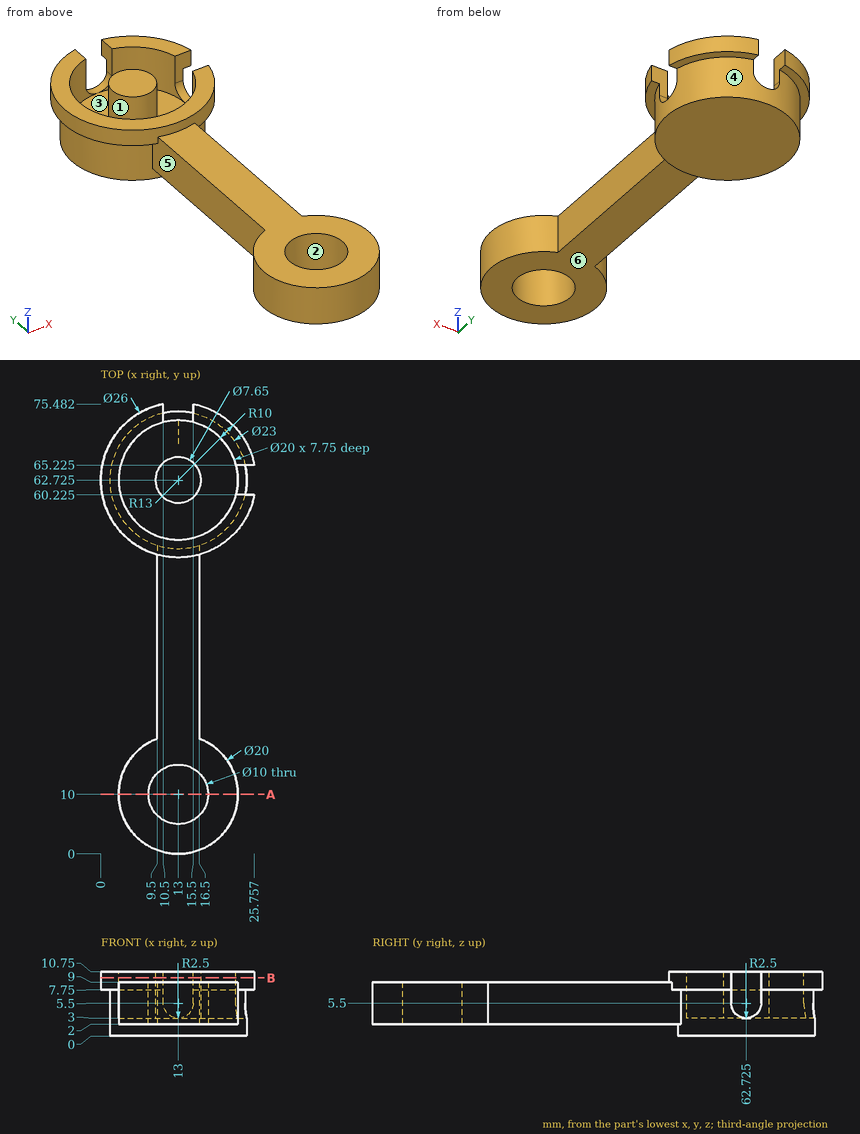
Input: dimensioned drawing with shaded views. Units: mm. Origin: part minimum x, y, z. A direction names the side the tool comes from. Give positions to 0.01 mm unless a question says otherwise; leave off trailing zeros. Write each loop counter-clockwise with the first axis right and the second up, starting at its lowest first coordinate (ties: lowest second). Pieces come first, ordered by that corner, then holes. Notation, with made-up numbers: (4, 88.25) - (52, 88.25) arc R15 ccw to (52, 109.25) - close; hole circle Ø2 at (60, 68). An arc over 180 degrees is marked (long way). One line per item, written item: value. Start each with the question number.
Q1. Material intervals for probe 1 along Y at (x, z) = (4.5, 4.75) (1 decimal); probe 2 along X at (y, z) = (28, 4); probe 3 along Y at (x, z) = (11, 4.5) (1 decimal), sorted ascending. Write a range as from..to.
Q2. First-contact query: pin 1 Ø3.5 at (y, z) = (30, 5.5) entering from -X; pin 2 Ø1.5 at (x, y) = (11, 46) entering from -Z; pin 3 Ø3 at (y, z) = (67, 5.5) entering from -X; pin 4 Ø6 at (x, y) = (15.5, 67) entering from +Z. Flat tips, straight axial feed; report the tip coordinate or a pass-through.
Q3. Section query A-A, the plane y = 10. Return the cut outline in (x, z), then the cut area to 3 significant figures.
Q4. Draft query along X for the marked faces 3, 4, 5 and 6. Return one class per face: +X half, -X half, draft (parallel to the pull), parting line (faces both ways), or undercut.
Q5. Set-up query: the marked faces 1 and 2. Return all of +Z, -Z, +X, -X, +Y, -Y with unobstructed straight access to the full face (end or side cutting, diameter ignored); none if empty.
Q6. Section query B-B, the plane z = 9.75. Count the separate pieces of the cut face and the enclosed holes in it.
Answer:
1. probe 1: y = 4.7..15.3, 55..57.5, 68..70.5
1. probe 2: x = 9.5..16.5
1. probe 3: y = 0.2..5.4, 14.6..52.9, 59.5..66
2. pin 1: stops at x = 9.5
2. pin 2: stops at z = 2
2. pin 3: stops at x = 1.84
2. pin 4: stops at z = 10.75
3. outline: (3, 2) - (8, 2) - (8, 9) - (3, 9) - close; (18, 2) - (23, 2) - (23, 9) - (18, 9) - close
3. area: 70.0 mm2
4. face 3: undercut
4. face 4: parting line
4. face 5: -X half
4. face 6: draft
5. face 1: +Z
5. face 2: +Z, -Z
6. separate pieces: 3
6. enclosed holes: 0
